Job drawing, mm, ordinate dimensions from the low corner. One solid piece. A direction names the side the tool comes from. Round coordinates to 2 decimals unless told otherwise and drop trailing zeros. Order: outer loops, then holes, each group sorted by start corner. A loop starts at its lowest first (then second) coordinate and runs counter-clockwise, first axis right, second up. Notation, with made-up numbers: (-23, 83) -> (3, 83) arc R11 cw to (3, 98) -> close; hole circle Ø11 at (75, 89). An arc over 180 degrees is marked (long way). Write item = value, one per line.
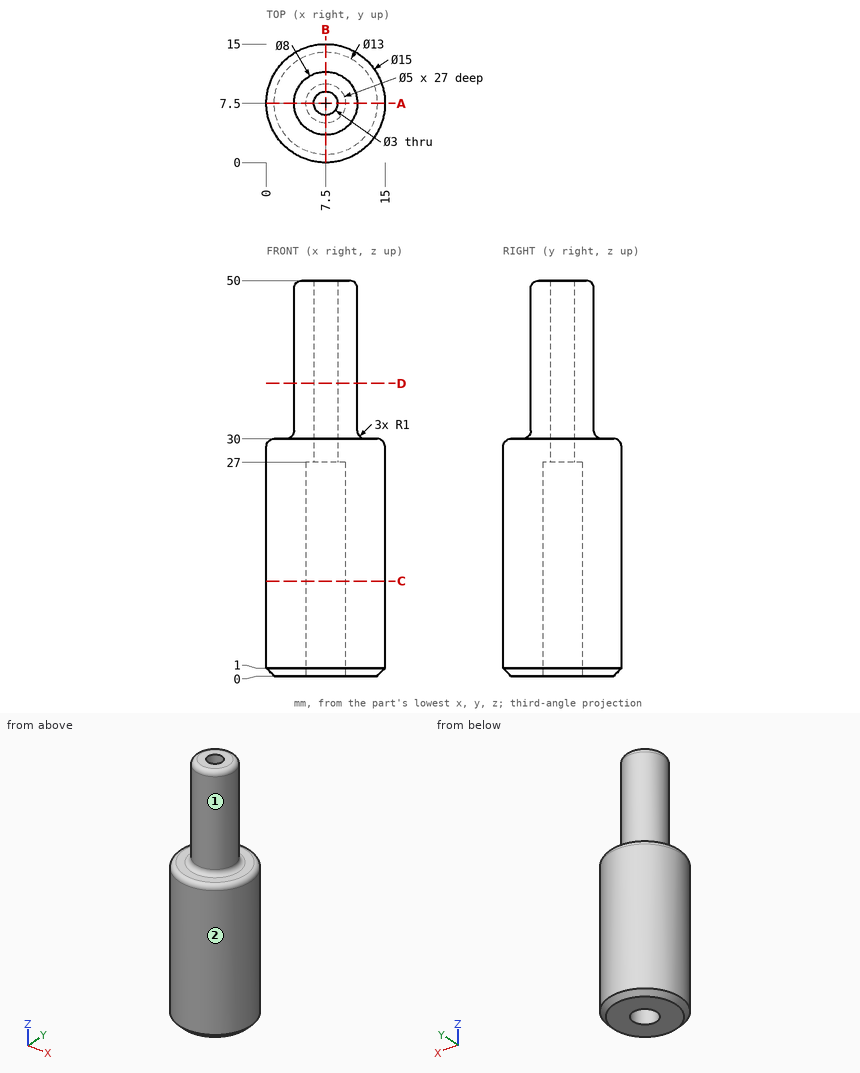
Q1. Cut at A-A, the plane y = 7.5. List the corners of the cut face in (x, z).
Check values:
outline = (0, 1) -> (1, 0) -> (5, 0) -> (5, 27) -> (6, 27) -> (6, 50) -> (4.5, 50) arc R1 ccw to (3.5, 49) -> (3.5, 31) arc R1 cw to (2.5, 30) -> (1, 30) arc R1 ccw to (0, 29) -> close; (9, 27) -> (10, 27) -> (10, 0) -> (14, 0) -> (15, 1) -> (15, 29) arc R1 ccw to (14, 30) -> (12.5, 30) arc R1 cw to (11.5, 31) -> (11.5, 49) arc R1 ccw to (10.5, 50) -> (9, 50) -> close
Q2. Probe probe 1 along X at (y, z) = (7.5, 32.5); probe 2 along X at (y, z) = (7.5, 17.5); probe 3 along Z at (x, y) = (13.25, 5.75). List the from-to ranges inside material, lowest first.
Check values:
probe_1 = 3.5 to 6, 9 to 11.5
probe_2 = 0 to 5, 10 to 15
probe_3 = 0 to 30
Q3. Flat gauge pins, fed straight in: pin 1 (5 mm diameter, centred on y = 12.5, z = 8, fed in from -X); pin 2 (4 mm diameter, centred on y = 5, z = 27, fed in from +X); pin 3 (2.5 mm diameter, centred on x = 8, y = 8.5, fed in from -Z). Where does each tip first touch, or does it go through?
Check values:
pin_1 = 0.43
pin_2 = 14.98
pin_3 = 27
Q4. Cut at D-D, the plane z = 37. List the corners of the cut face in (x, y), and give its area (3 significant figures).
Check values:
outline = circle Ø8 at (7.5, 7.5); hole circle Ø3 at (7.5, 7.5)
area = 43.2 mm²
Q5. Which spindle directions (+Z, -Z, +X, -X, +Y, -Y) get a long thin tool onto all of the face, cutting with end or side? Do the marked faces 1 and 2. Say none if no direction does.
Check values:
face_1 = +Z
face_2 = +Z, -Z
Q6. Cut at C-C, the plane z = 12. List the corners of the cut face in (x, y).
Check values:
outline = circle Ø15 at (7.5, 7.5); hole circle Ø5 at (7.5, 7.5)
